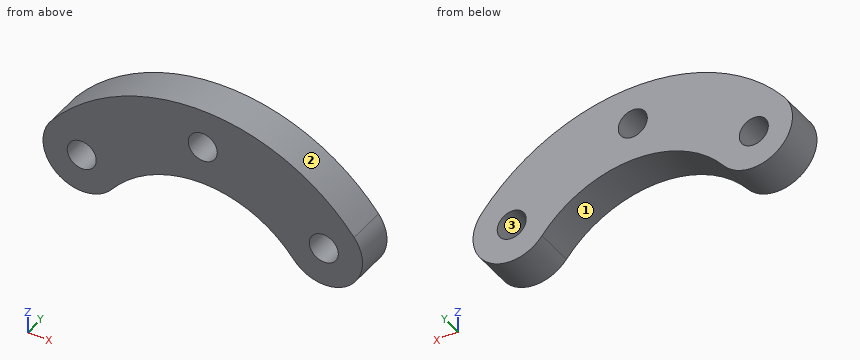
```python
from build123d import *

# Parameters (mm, degrees)
SKETCH1_R           = 1.5
BOSS_EXTRUDE1_DEPTH = 4


with BuildPart() as part:
    # Sketch1 → Boss-Extrude1 (new body)
    with BuildSketch(Plane(origin=(0, 0, 0), x_dir=(1, 0, 0), z_dir=(0, 1, 0))):
        with BuildLine():
            ThreePointArc((-9.375, -7.490619133), (0, -12), (9.375, -7.490619133))
            ThreePointArc((9.375, -7.490619133), (14.996873044, -6.862492178), (15.625, -12.484365222))
            ThreePointArc((15.625, -12.484365222), (0, -20), (-15.625, -12.484365222))
            ThreePointArc((-15.625, -12.484365222), (-14.996873044, -6.862492178), (-9.375, -7.490619133))
        make_face()
        with Locations((-12.5, -9.987492178)):
            Circle(SKETCH1_R, mode=Mode.SUBTRACT)
        with Locations((12.5, -9.987492178)):
            Circle(SKETCH1_R, mode=Mode.SUBTRACT)
        with Locations((0, -16)):
            Circle(SKETCH1_R, mode=Mode.SUBTRACT)
    extrude(amount=BOSS_EXTRUDE1_DEPTH)


solid = part.part
```
Source: CAD feature listing. Evaluate the final solid. Frame: model axes, mm. Face numbers are marked on the shaded views. Give positions to 0.01 mm unless a question says otherwise; leave off trailing zeros. Loops run counter-clockwise (first coordinate to the right, second up) from the corner with the lowest first, then second, coordinate; pieces in that order, holes last. Notation, with made-up numbers: (76, 71.25) - (90, 71.25) arc R12 cw to (90, 85.25) - close; hole circle Ø5 at (38.25, 75). An arc over 180 degrees is marked (long way). Use CSV: the item, a comma, the result in double quotes. Start each with the question number.
1. Section B-B (x = -13). Output: boundary loops of the cut face in (y, z).
2. Draft query along Z for the marked faces 1, 2 and 3. Return one class per face: +Z half, -Z half, draft (parallel to the pull), parting line (faces both ways), or undercut.
3. Section C-C (y = 0.4). Output: boundary loops of the cut face in (x, z) (1 decimal), then the cut area to 3 significant figures.
4. Pin query (flat end, axial travel): pin 1 (2.5 mm diameter, centred on x = 12.5, z = 9.99, fed in from -Y); pin 2 (4 mm diameter, centred on x = -12.5, z = 9.99, fed in from -Y); pin 3 (2 mm diameter, centred on x = -2.5, y = 1.5, fed in from -Z); pin 4 (1 mm diameter, centred on x = 6.5, y = 1, fed in from +Z). Return the tip coordinate at first contact, or that it passes through.
5. Ray query, L1, parallel to X at y = 2.8, z = 9.75; L2, parallel to Z at x = 12.5, y = 1.1; L3, parallel to X at y = 0.85, z = 10.25. Return the intervals inside material, ascending.
6. Section D-D (z = 11). Output: boundary loops of the cut face in (x, y), then the cut area to 3 significant figures.
7. Section A-A (z = 16). Output: boundary loops of the cut face in (x, y), then the cut area to 3 significant figures.
Response:
1,outline,"(0, 6.02) - (4, 6.02) - (4, 8.57) - (0, 8.57) - close; (0, 11.4) - (4, 11.4) - (4, 15.2) - (0, 15.2) - close"
2,face 1,"-Z half"
2,face 2,"+Z half"
2,face 3,"undercut"
3,outline,"(-15.6, 12.5) arc R4 ccw to (-9.4, 7.5) arc R12 cw to (9.4, 7.5) arc R4 ccw to (15.6, 12.5) arc R20 ccw to start; hole circle Ø3 at (-12.5, 10); hole circle Ø3 at (0, 16); hole circle Ø3 at (12.5, 10)"
3,area,"259 mm²"
4,pin 1,"through"
4,pin 2,"y = 0"
4,pin 3,"z = 11.48"
4,pin 4,"z = 19.08"
5,L1,"-16.49 to -13.98, -11.02 to -7, 7 to 11.02, 13.98 to 16.49"
5,L2,"5.99 to 8.49, 11.49 to 15.61"
5,L3,"-16.49 to -13.98, -11.02 to -6.24, 6.24 to 11.02, 13.98 to 16.49"
6,outline,"(-16.37, 0) - (-13.61, 0) - (-13.61, 4) - (-16.37, 4) - close; (-11.39, 0) - (-4.8, 0) - (-4.8, 4) - (-11.39, 4) - close; (4.8, 0) - (11.39, 0) - (11.39, 4) - (4.8, 4) - close; (13.61, 0) - (16.37, 0) - (16.37, 4) - (13.61, 4) - close"
6,area,"74.9 mm²"
7,outline,"(-12, 0) - (-1.5, 0) - (-1.5, 4) - (-12, 4) - close; (1.5, 0) - (12, 0) - (12, 4) - (1.5, 4) - close"
7,area,"84.0 mm²"
